Check sheet for the modelled part. Datum: model origin and axes. Units: mm. Give positions to 0.01 mm unless a question says otherwise; leave off trailing zeros. Write each loop counter-clockwise with the first axis right and the second up, starting at its lowest first coordinate (ties: lowest second). Pieces come first, ordered by that corner, then holes.
from build123d import *
from build123d.topology import SkipClean

# Parameters (mm, degrees)
SKETCH1_W                      = 390
SKETCH1_H                      = 3
BOSS_EXTRUDE1_DEPTH            = 5
DRAFT1_ANGLE                   = -15
CIRPATTERN1_COUNT              = 12
DRAFT1_OF_CIRPATTERN1_2_ANGLE  = -15
DRAFT1_OF_CIRPATTERN1_3_ANGLE  = -15
DRAFT1_OF_CIRPATTERN1_4_ANGLE  = -15
DRAFT1_OF_CIRPATTERN1_5_ANGLE  = -15
DRAFT1_OF_CIRPATTERN1_6_ANGLE  = -15
DRAFT1_OF_CIRPATTERN1_7_ANGLE  = -15
DRAFT1_OF_CIRPATTERN1_8_ANGLE  = -15
DRAFT1_OF_CIRPATTERN1_9_ANGLE  = -15
DRAFT1_OF_CIRPATTERN1_10_ANGLE = -15
DRAFT1_OF_CIRPATTERN1_11_ANGLE = -15
DRAFT1_OF_CIRPATTERN1_12_ANGLE = -15
SKETCH3_OUTSIDE_W              = 265.338
SKETCH3_OUTSIDE_H              = 265.338
CUT_EXTRUDE1_DEPTH             = 563.983125857


# Read off the part's stored shape, not the designer's step: CSK for M4 Countersunk Flat Head Screw1
with BuildPart() as part:
    # Sketch1 → Revolve1 (revolve)
    with BuildSketch(Plane.XY, mode=Mode.PRIVATE) as revolve1_sk:
        with Locations((355, 83.5)):
            Rectangle(SKETCH1_W, SKETCH1_H)
    revolve(revolve1_sk.sketch.rotate(Axis((0, 0, 0), (1, 0, 0)), 90), axis=Axis((0, 0, 0), (1, 0, 0)))

    # Sketch2 → Boss-Extrude1 (add, symmetric)
    with BuildSketch(Plane(origin=(155, 0, 0), x_dir=(0, 0, -1), z_dir=(1, 0, 0))):
        with BuildLine():
            Line((10.703147762, 81.298478633), (11.094726339, 84.272813217))
            ThreePointArc((11.094726339, 84.272813217), (0, 85), (-11.094726339, 84.272813217))
            Line((-11.094726339, 84.272813217), (-10.703147762, 81.298478633))
            ThreePointArc((-10.703147762, 81.298478633), (0, 82), (10.703147762, 81.298478633))
        make_face()
    boss_extrude1 = extrude(amount=BOSS_EXTRUDE1_DEPTH, both=True)

    # Draft1
    draft1_faces = [part.faces().sort_by_distance(p)[0] for p in [
        (155, 82.785645925, 10.89893705),
        (155, 82.785645925, -10.89893705),
    ]]
    draft(draft1_faces, Plane(origin=(155, 0, 0), x_dir=(0, 0, 1), z_dir=(1, 0, 0)), DRAFT1_ANGLE)

    # CirPattern1: Boss-Extrude1 ×12 about axis
    with SkipClean():  # the faces are left unmerged after this step: merging them gives an invalid solid
        cirpattern1_axis = Axis((0, 0, 0), (1, 0, 0))
        for i in range(1, CIRPATTERN1_COUNT):
            add(boss_extrude1.rotate(cirpattern1_axis, i * 360 / CIRPATTERN1_COUNT))

    # Draft1 of CirPattern1 2
    draft1_of_cirpattern1_2_faces = [part.faces().sort_by_distance(p)[0] for p in [
        (155, 66.245003914, 50.831579322),
        (155, 77.143940965, 31.954066602),
    ]]
    draft(draft1_of_cirpattern1_2_faces, Plane(origin=(155, 0, 0), x_dir=(0, -0.49999999999999994, 0.8660254037844387), z_dir=(1, 0, 0)), DRAFT1_OF_CIRPATTERN1_2_ANGLE)

    # Draft1 of CirPattern1 3
    draft1_of_cirpattern1_3_faces = [part.faces().sort_by_distance(p)[0] for p in [
        (155, 31.954066602, 77.143940965),
        (155, 50.831579322, 66.245003914),
    ]]
    draft(draft1_of_cirpattern1_3_faces, Plane(origin=(155, 0, 0), x_dir=(0, -0.8660254037844386, 0.5000000000000001), z_dir=(1, 0, 0)), DRAFT1_OF_CIRPATTERN1_3_ANGLE)

    # Draft1 of CirPattern1 4
    draft1_of_cirpattern1_4_faces = [part.faces().sort_by_distance(p)[0] for p in [
        (155, -10.89893705, 82.785645925),
        (155, 10.89893705, 82.785645925),
    ]]
    draft(draft1_of_cirpattern1_4_faces, Plane(origin=(155, 0, 0), x_dir=(0, -1, 0), z_dir=(1, 0, 0)), DRAFT1_OF_CIRPATTERN1_4_ANGLE)

    # Draft1 of CirPattern1 5
    draft1_of_cirpattern1_5_faces = [part.faces().sort_by_distance(p)[0] for p in [
        (155, -50.831579322, 66.245003914),
        (155, -31.954066602, 77.143940965),
    ]]
    draft(draft1_of_cirpattern1_5_faces, Plane(origin=(155, 0, 0), x_dir=(0, -0.8660254037844387, -0.4999999999999998), z_dir=(1, 0, 0)), DRAFT1_OF_CIRPATTERN1_5_ANGLE)

    # Draft1 of CirPattern1 6
    draft1_of_cirpattern1_6_faces = [part.faces().sort_by_distance(p)[0] for p in [
        (155, -77.143940965, 31.954066602),
        (155, -66.245003914, 50.831579322),
    ]]
    draft(draft1_of_cirpattern1_6_faces, Plane(origin=(155, 0, 0), x_dir=(0, -0.49999999999999994, -0.8660254037844387), z_dir=(1, 0, 0)), DRAFT1_OF_CIRPATTERN1_6_ANGLE)

    # Draft1 of CirPattern1 7
    draft1_of_cirpattern1_7_faces = [part.faces().sort_by_distance(p)[0] for p in [
        (155, -82.785645925, -10.89893705),
        (155, -82.785645925, 10.89893705),
    ]]
    draft(draft1_of_cirpattern1_7_faces, Plane(origin=(155, 0, 0), x_dir=(0, 0, -1), z_dir=(1, 0, 0)), DRAFT1_OF_CIRPATTERN1_7_ANGLE)

    # Draft1 of CirPattern1 8
    draft1_of_cirpattern1_8_faces = [part.faces().sort_by_distance(p)[0] for p in [
        (155, -66.245003914, -50.831579322),
        (155, -77.143940965, -31.954066602),
    ]]
    draft(draft1_of_cirpattern1_8_faces, Plane(origin=(155, 0, 0), x_dir=(0, 0.5000000000000001, -0.8660254037844386), z_dir=(1, 0, 0)), DRAFT1_OF_CIRPATTERN1_8_ANGLE)

    # Draft1 of CirPattern1 9
    draft1_of_cirpattern1_9_faces = [part.faces().sort_by_distance(p)[0] for p in [
        (155, -31.954066602, -77.143940965),
        (155, -50.831579322, -66.245003914),
    ]]
    draft(draft1_of_cirpattern1_9_faces, Plane(origin=(155, 0, 0), x_dir=(0, 0.8660254037844384, -0.5000000000000004), z_dir=(1, 0, 0)), DRAFT1_OF_CIRPATTERN1_9_ANGLE)

    # Draft1 of CirPattern1 10
    draft1_of_cirpattern1_10_faces = [part.faces().sort_by_distance(p)[0] for p in [
        (155, 10.89893705, -82.785645925),
        (155, -10.89893705, -82.785645925),
    ]]
    draft(draft1_of_cirpattern1_10_faces, Plane.YZ.offset(155), DRAFT1_OF_CIRPATTERN1_10_ANGLE)

    # Draft1 of CirPattern1 11
    draft1_of_cirpattern1_11_faces = [part.faces().sort_by_distance(p)[0] for p in [
        (155, 50.831579322, -66.245003914),
        (155, 31.954066602, -77.143940965),
    ]]
    draft(draft1_of_cirpattern1_11_faces, Plane(origin=(155, 0, 0), x_dir=(0, 0.8660254037844386, 0.5000000000000001), z_dir=(1, 0, 0)), DRAFT1_OF_CIRPATTERN1_11_ANGLE)

    # Draft1 of CirPattern1 12
    draft1_of_cirpattern1_12_faces = [part.faces().sort_by_distance(p)[0] for p in [
        (155, 77.143940965, -31.954066602),
        (155, 66.245003914, -50.831579322),
    ]]
    draft(draft1_of_cirpattern1_12_faces, Plane(origin=(155, 0, 0), x_dir=(0, 0.5000000000000004, 0.8660254037844384), z_dir=(1, 0, 0)), DRAFT1_OF_CIRPATTERN1_12_ANGLE)

    # Sketch3 outside → Cut-Extrude1 (cut, through all)
    with SkipClean():  # the faces are left unmerged after this step: merging them gives an invalid solid
        with BuildSketch(Plane(origin=(0, 0, 0), x_dir=(0, 0, -1), z_dir=(1, 0, 0))):
            Rectangle(SKETCH3_OUTSIDE_W, SKETCH3_OUTSIDE_H)
            with BuildLine():
                Line((0, 0), (-85, 0))
                ThreePointArc((-85, 0), (0, 85), (85, 0))
                Line((85, 0), (0, 0))
            make_face(mode=Mode.SUBTRACT)
        extrude(amount=CUT_EXTRUDE1_DEPTH, mode=Mode.SUBTRACT)

    # CSK for M4 Countersunk Flat Head Scr 2 → CSK for M4 Countersunk Flat Head Screw1 (revolve, cut)
    with SkipClean():  # the faces are left unmerged after this step: merging them gives an invalid solid
        with BuildSketch(Plane(origin=(540, 0, 0), x_dir=(1, 0, 0), z_dir=(0, 0, 1))):
            Polygon((4.700033545, 85.000033545), (0, 85.000033545), (0, 81.96910869), (2.25, 81.96910869), (2.25, 82.55), align=None)
        revolve(axis=Axis((540, 0, 0), (0, 1, 0)), mode=Mode.SUBTRACT)

    # CSK for M4 Countersunk Flat Head Scr 3 o → CSK for M4 Countersunk Flat Head Scr 3 (revolve, cut)
    with SkipClean():  # the faces are left unmerged after this step: merging them gives an invalid solid
        with BuildSketch(Plane(origin=(540, 0, 0), x_dir=(1, 0, 0), z_dir=(0, -1, 0))):
            Polygon((0, -85.000002015), (4.700002015, -85.000002015), (2.25, -82.55), (2.25, -81.969112603), (0, -81.969112603), align=None)
            Polygon((0, 81.969112603), (2.25, 81.969112603), (2.25, 82.55), (4.700002015, 85.000002015), (0, 85.000002015), align=None)
        revolve(axis=Axis((540, 0, 0), (0, 0, 1)), mode=Mode.SUBTRACT)


solid = part.part
1) Gauge pin test, flat ends, axial feed: pin 1 (2 mm diameter, centred on x = 300, z = 20.5, fed in from +Y); pin 2 (6.5 mm diameter, centred on y = 21.5, z = 82, fed in from -X); pin 3 (10 mm diameter, centred on x = 361, y = 19, fed in from -Z); pin 4 (6 mm diameter, centred on y = 72, z = -54.5, fed in from +X). Record the tip position at first contact, or that the pin passes through.
2) Sectioned sample at B-B on x = 290. Record the boundary of the cut face in (y, z), then the cut area to 3 significant figures.
3) Draft check along Z on faces 1 (the conical face through (541.11, 82.7, 2.13)), 2 (the flat face through (550, 83, 0)). Enter one of: +Z half, -Z half, draft (parallel to the pull), parting line (faces both ways), or undercut.
4) Scan lines: L1, parallel to X at y = 82.4, z = 0; L2, parallel to Z at x = 202, y = 33; L3, parallel to Z at x = 295, y = 25.5. Record each from-to range of solid material in increasing order.
5) Sectioned sample at A-A on y = 25. Record the boundary of the cut face in (x, z), then the cut area to 3 significant figures.
Answers below:
1. pin 1: stops at y = 82.73
1. pin 2: stops at x = 160
1. pin 3: stops at z = -83.84
1. pin 4: passes through
2. outline: (0, -85) arc R85 ccw to (0, 85) - (0, 82) arc R82 cw to (0, -82) - close
2. area: 787 mm2
3. face 1: undercut
3. face 2: draft
4. L1: x = 150 to 537.75, 542.25 to 550
4. L2: z = -78.33 to -75.07, 75.07 to 78.33
4. L3: z = -81.08 to -77.93, 77.93 to 81.08
5. outline: (160, -81.24) - (550, -81.24) - (550, -78.1) - (160, -78.1) - close; (160, 78.1) - (550, 78.1) - (550, 81.24) - (160, 81.24) - close
5. area: 2,450 mm2
